Verification items for the finished model (mm, model axes). Face numbers are marked on the shaded views. A direction names the side the tool comes from. Round coordinates to 2 decimals unless told otherwise and drop trailing zeros. Write each loop counter-clockwise with the first axis right and the second up, starting at its lowest first coordinate (ties: lowest second). Pieces come first, ordered by that corner, then holes. Notation, with made-up numbers: (25.25, 42.5) - (29.25, 42.5) arc R25 cw to (29.25, 55.5) - close; hole circle Ø1 at (11.5, 50). An arc over 180 degrees is marked (long way). Answer as a JSON object with one key per item and string values.
```python
from build123d import *

# Parameters (mm, degrees)
BOSS_EXTRUDE1_DEPTH  = 12.5
BOSS_EXTRUDE2_DEPTH  = 2.5
FILLET1_R            = 2
M3_CLEARANCE_HOLE1_D = 3.2


with BuildPart() as part:
    # Sketch1 → Boss-Extrude1 (new, symmetric)
    with BuildSketch(Plane(origin=(0, 0, 0), x_dir=(0, 0, -1), z_dir=(1, 0, 0))):
        with BuildLine():
            Line((-7.5, 9.367496998), (-7.5, 14))
            Line((-7.5, 14), (7.5, 14))
            Line((7.5, 14), (7.5, 9.367496998))
            ThreePointArc((7.5, 9.367496998), (0, 12), (-7.5, 9.367496998))
        make_face()
    extrude(amount=BOSS_EXTRUDE1_DEPTH, both=True)

    # Sketch2 → Boss-Extrude2 (add, symmetric)
    with BuildSketch(Plane(origin=(0, 0, 0), x_dir=(0, 0, -1), z_dir=(1, 0, 0))):
        with BuildLine():
            Line((-5, 14), (-3, 14))
            ThreePointArc((-3, 14), (0, 17), (3, 14))
            Line((3, 14), (5, 14))
            ThreePointArc((5, 14), (0, 19), (-5, 14))
        make_face()
    extrude(amount=BOSS_EXTRUDE2_DEPTH, both=True)

    # Fillet1
    fillet1_edges = [part.edges().sort_by_distance(p)[0] for p in [
        (0, 14, -5),
        (0, 14, 5),
    ]]
    fillet(fillet1_edges, radius=FILLET1_R)
    fillet1_2_edges = [part.edges().sort_by_distance(p)[0] for p in [
        (12.5, 11.683748499, 7.5),
        (-12.5, 11.683748499, 7.5),
        (-12.5, 11.683748499, -7.5),
        (12.5, 11.683748499, -7.5),
    ]]
    fillet(fillet1_2_edges, radius=FILLET1_R)

    # M3 Clearance Hole1 (through all)
    with Locations(Plane(origin=(0, 14, 0), x_dir=(1, 0, 0), z_dir=(0, 1, 0))):
        with Locations((-7.5, 0), (7.5, 0)):
            Hole(M3_CLEARANCE_HOLE1_D / 2)


solid = part.part
```
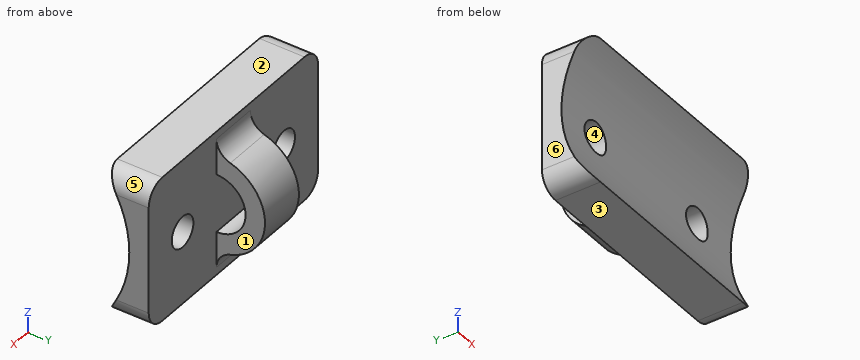
Q1. Section check D-D, the plane z = 0. Record the cut outline in (x, y), then the cut area to 3 significant figures.
Geometry check:
{"outline": "(-12.5, 12) - (-9.1, 12) - (-9.1, 14) - (-12.5, 14) - close; (-5.9, 12) - (5.9, 12) - (5.9, 14) - (-5.9, 14) - close; (-2.5, 17) - (2.5, 17) - (2.5, 19) - (-2.5, 19) - close; (9.1, 12) - (12.5, 12) - (12.5, 14) - (9.1, 14) - close", "area": "47.2 mm2"}
Q2. Section check B-B, the plane y = 12.75. Record the cut outline in (x, z), then the cut area to 3 significant figures.
Geometry check:
{"outline": "(-12.5, -5.5) arc R2 ccw to (-10.5, -7.5) - (10.5, -7.5) arc R2 ccw to (12.5, -5.5) - (12.5, 5.5) arc R2 ccw to (10.5, 7.5) - (-10.5, 7.5) arc R2 ccw to (-12.5, 5.5) - close; hole circle Ø3.2 at (-7.5, 0); hole circle Ø3.2 at (7.5, 0)", "area": "355 mm2"}
Q3. Material ranges on line 1 along Z through (x, y) = (-7.5, 12.3); line 2 along Y through (x, z) = (-2.25, 0); line 3 along Z through (x, y) = (7, 10), recorded low to high. Write a range as [from, to].
Geometry check:
{"line 1": "z = [-7.5, -1.6], [1.6, 7.5]", "line 2": "y = [12, 14], [17, 19]", "line 3": "z = [-7.5, -6.63], [6.63, 7.5]"}
Q4. Release check for a two-part mould opening along Z. For the marked faces 3, 4, 5 and 6 record: released by +Z, released by -Z, zero draft, split by the parting line, or undercut.
Geometry check:
{"face 3": "released by -Z", "face 4": "undercut", "face 5": "released by +Z", "face 6": "zero draft"}
Q5. Set-up check for the marked faces 1 and 2: record each of +Z, -Z, +X, -X, +Y, -Y from which the full face is reachable in a straight line by a thin tool's end or side.
Geometry check:
{"face 1": "+Z, -Z, +X, +Y", "face 2": "+Z, +X, -X, +Y, -Y"}
Q6. Gauge pin test, flat ends, axial feed: P1, Ø4, axis at y = 16.5, z = -1.5, coming from the -X side; P2, Ø2, axis at x = 9.5, z = -3, coming from the -Y side; P3, Ø1.5, axis at x = -4.5, z = -3, coming from the -Y side. Record the tip position at first contact, or that the pin passes through.
Geometry check:
{"P1": "stops at x = -2.5", "P2": "stops at y = 11.31", "P3": "stops at y = 11.4"}
Q7. Section check A-A, the plane x = -7.5. Record the cut outline in (y, z), then the cut area to 3 significant figures.
Geometry check:
{"outline": "(9.37, -7.5) - (14, -7.5) - (14, -1.6) - (11.89, -1.6) arc R12 cw to start; (9.37, 7.5) arc R12 cw to (11.89, 1.6) - (14, 1.6) - (14, 7.5) - close", "area": "36.0 mm2"}
Q8. Section check C-C, the plane x = 0.5. Record the cut outline in (y, z).
Geometry check:
{"outline": "(9.37, -7.5) - (14, -7.5) - (14, -6.71) arc R2 cw to (15.43, -4.79) arc R5 ccw to (15.43, 4.79) arc R2 cw to (14, 6.71) - (14, 7.5) - (9.37, 7.5) arc R12 cw to start; hole (14, -3) arc R3 ccw to (14, 3) - close"}
